```python
from build123d import *

# Parameters (mm, degrees)
SKETCH1_R           = 8
BOSS_EXTRUDE1_DEPTH = 36.5
CHAMFER1_SIZE       = 2
SKETCH2_R           = 11.75
BOSS_EXTRUDE2_DEPTH = 5


with BuildPart() as part:
    # Sketch1 → Boss-Extrude1 (new body)
    with BuildSketch(Plane(origin=(0, 0, 0), x_dir=(1, 0, 0), z_dir=(0, 1, 0))):
        Circle(SKETCH1_R)
    extrude(amount=BOSS_EXTRUDE1_DEPTH)

    # Chamfer1
    chamfer1_edges = [part.edges().sort_by_distance(p)[0] for p in [
        (-8, 0, 0),
    ]]
    chamfer(chamfer1_edges, length=CHAMFER1_SIZE)

    # Sketch2 → Boss-Extrude2 (add)
    with BuildSketch(Plane(origin=(0, 36.5, 0), x_dir=(1, 0, 0), z_dir=(0, 1, 0))):
        Circle(SKETCH2_R)
    extrude(amount=BOSS_EXTRUDE2_DEPTH)


solid = part.part
```
Part model, mm, in its own coordinate system. A direction names the side the tool comes from. Round coordinates to 2 decimals unless told otherwise and drop trailing zeros. Loops run counter-clockwise (first coordinate to the right, second up) from the corner with the lowest first, then second, coordinate; pieces in that order, holes last. Notation, with made-up numbers: (82, -32.75) -> (135, -32.75) arc R15 cw to (135, -5.75) -> close; hole circle Ø1 at (-24, 32). An arc over 180 degrees is marked (long way). Use one line per item in the form item = value. Start each with the question number.
Item 1: Drop flat-ended pins along their axis: pin 1 Ø3 at (x, z) = (-6.5, -8.5) entering from -Y; pin 2 Ø8 at (y, z) = (23, -4.5) entering from +X; pin 3 Ø3 at (x, y) = (2.5, 15.5) entering from -Z. Give the stop position or say it passes through.
Item 2: Band-saw the part on B-B (z = 0). List the corners of the cut face in (x, y).
Item 3: Drill centre lines: line 1 along Y through (x, z) = (-4.25, 9.75); line 2 along X through (y, z) = (20, 0); line 3 along Z through (x, y) = (-6.25, 29). Where is each one in solid material? Low to high.
Item 4: Band-saw the part on C-C (y = 11.5). List the corners of the cut face in (x, z).
Item 5: Band-saw the part on D-D (x = -8.5). List the corners of the cut face in (y, z), plus the area to 3 significant figures.
Item 6: Band-saw the part on A-A (x = 0). List the corners of the cut face in (y, z).
Item 7: Tool access for faces 1 (the flat face through (0, 0, 0)), 2 (the cylindrical face through (-1.73, 19.01, 7.81)): list every direction of +Z, -Z, +X, -X, +Y, -Y with a clear straight run to the whole face (end or side of a thin tool).
Data:
q1.pin_1 = 36.5
q1.pin_2 = 7.98
q1.pin_3 = -7.94
q2.outline = (-11.75, 36.5) -> (-8, 36.5) -> (-8, 2) -> (-6, 0) -> (6, 0) -> (8, 2) -> (8, 36.5) -> (11.75, 36.5) -> (11.75, 41.5) -> (-11.75, 41.5) -> close
q3.line_1 = 36.5 to 41.5
q3.line_2 = -8 to 8
q3.line_3 = -4.99 to 4.99
q4.outline = circle Ø16 at (0, 0)
q5.outline = (36.5, -8.11) -> (41.5, -8.11) -> (41.5, 8.11) -> (36.5, 8.11) -> close
q5.area = 81.1 mm^2
q6.outline = (0, -6) -> (2, -8) -> (36.5, -8) -> (36.5, -11.75) -> (41.5, -11.75) -> (41.5, 11.75) -> (36.5, 11.75) -> (36.5, 8) -> (2, 8) -> (0, 6) -> close
q7.face_1 = +Z, -Z, +X, -X, -Y
q7.face_2 = -Y
